Part print with two shaded views. Sizes in mm from the minimum x, y, z corner. A direction names the side the tool comes from. Give positions to 0.01 mm unless a question says otherwise; leave off trailing zeros. Loops run counter-clockwise (first coordinate to the right, second up) from the corner with the lowest first, then second, coordinate; pieces in that order, holes last. Notation, with made-up numbers: M -17,55 L 27,55 A28 ccw 27,78 Z; hole C 12,54.5 d7. An arc over 180 degrees is marked long. Answer in a Markdown table with one row per item.
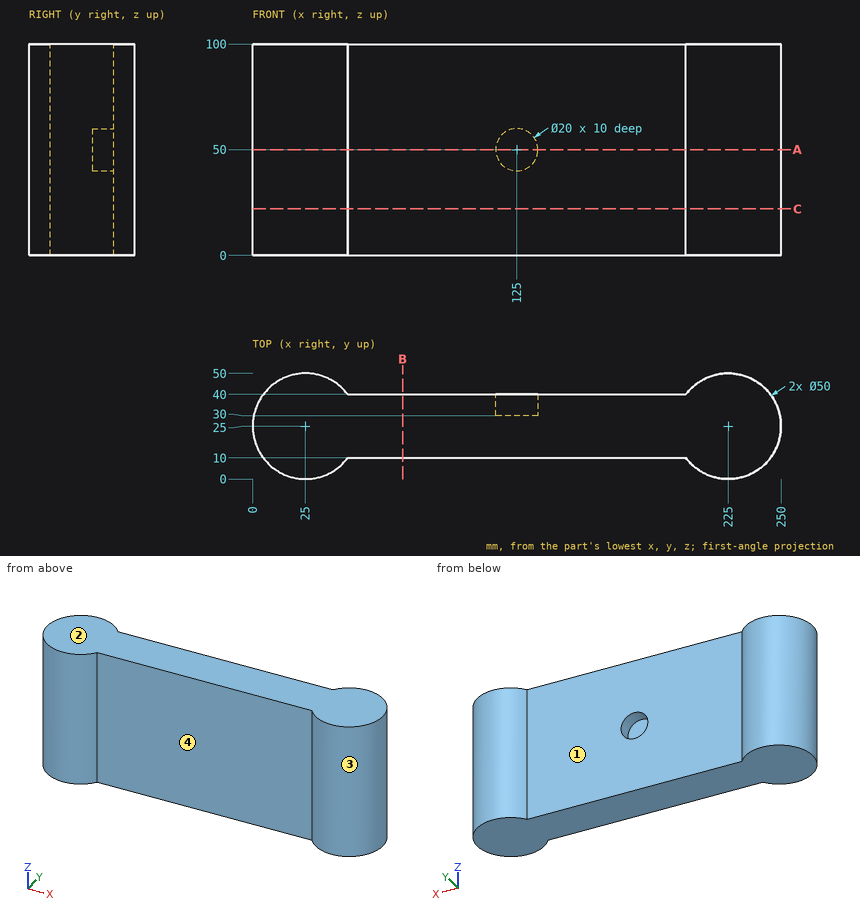
Q1. Probe probe 1 along Y at (x, z) = (179, 38); probe 2 along X at (y, z) = (25, 61.5); probe 3 along X at (y, z) = (8.5, 7). List the from-to ranges inside material, lowest first.
Reported:
| item | result |
|---|---|
| probe 1 | 10 to 40 |
| probe 2 | 0 to 250 |
| probe 3 | 6.22 to 43.78, 206.22 to 243.78 |
Q2. Saw through at A-A (z = 50). Give the cut face in (x, y).
Reported:
| item | result |
|---|---|
| outline | M 45,10 L 205,10 A25 ccw long 205,40 L 135,40 L 135,30 L 115,30 L 115,40 L 45,40 A25 ccw long Z |
Q3. Drop flat-ended pins along their axis: pin 1 (3 mm diameter, centred on x = 210, z = 22.5, fed in from -Y); pin 2 (8 mm diameter, centred on x = 191.5, z = 18.5, fed in from -Y); pin 3 (1 mm diameter, centred on x = 203.5, z = 23.5, fed in from +Y); pin 4 (12 mm diameter, centred on x = 99, y = 45, fed in from -Z). Give the stop position or say it passes through.
Reported:
| item | result |
|---|---|
| pin 1 | y = 3.96 |
| pin 2 | y = 10 |
| pin 3 | y = 40 |
| pin 4 | z = 0 |
Q4. 3-axis set-ups, long thin cutter, end or side, ignore diameter. For the marked faces 3 and 4: which of +Z, -Z, +X, -X, +Y, -Y reach the whole face in a straight line?
Reported:
| item | result |
|---|---|
| face 3 | +Z, -Z |
| face 4 | +Z, -Z, -Y |
Q5. Saw through at C-C (z = 22). Give the cut face in (x, y), and give its area (3 significant figures).
Reported:
| item | result |
|---|---|
| outline | M 45,10 L 205,10 A25 ccw long 205,40 L 45,40 A25 ccw long Z |
| area | 8,520 mm² |
Q6. Mould opens along X. For the marked faces 1 and 2 say: released by +X, released by -X, zero draft, split by the parting line, or undercut.
Reported:
| item | result |
|---|---|
| face 1 | undercut |
| face 2 | zero draft |
Q7. Saw through at B-B (x = 71). Give the cut face in (y, z), and give its area (3 significant figures).
Reported:
| item | result |
|---|---|
| outline | M 10,0 L 40,0 L 40,100 L 10,100 Z |
| area | 3,000 mm² |
